The model under review builds one solid part; all positions refer to its coordinate system, in mm. Face numbers are marked on the shaded views. A direction names the side the tool comes from. Round coordinates to 2 decimals unless told otherwise and drop trailing zeros. Loops run counter-clockwise (first coordinate to the right, second up) from the corner with the lowest first, then second, coordinate; pieces in that order, holes last. Notation, with made-up numbers: (-22.5, -10.75) -> (13.5, -10.75) arc R31 cw to (13.5, 21.25) -> close; hole circle Ø3 at (13.25, 2.5). An arc over 180 degrees is marked (long way). Use a Markdown table: item, result. Add a question column.
1) Wall thickness on probe 1 along Y at (x, z) = (4.5, 0); probe 2 along X at (y, z) = (-10, -8); probe 3 along Y at (x, z) = (9, 0): over which ranges is each line inside the solid? List them lowest first.
2) For the marked faces 1, 2 and 3, list the 3-axis set-ups (+Z, -Z, +X, -X, +Y, -Y) from which the entire face can be reached by the end or side of a thin tool; tool diameter is ignored.
3) Insertion check: pin 1 (13.5 mm diameter, centred on y = 1.5, z = 5.5, fed in from -X); pin 2 (1.5 mm diameter, centred on x = -14, z = -6, fed in from -Y); pin 3 (1 mm diameter, centred on x = 8, y = 3, fed in from +Z). Each pin has a flat end and moves straight along its axis. Give the tip position at first contact, or say it passes through.
4) Consider section A-A on x = 0. Give the boundary of the cut face in (y, z), plus the area to 3 significant figures.
5) Consider section B-B on x = -19.5. Give the boundary of the cut face in (y, z), plus the area to 3 significant figures.
6) Mouldability with a two-part tool opening along Y and no side actions: class the marked faces 4, 5 and 6 as released by +Y, released by -Y, zero draft, split by the parting line, or undercut.
7) Consider section C-C on x = 12. Give the boundary of the cut face in (y, z).
from build123d import *

# Parameters (mm, degrees)
EXTRUDE1_DEPTH     = 32.146875
SKETCH3_OUTSIDE_W  = 278.22
SKETCH3_OUTSIDE_H  = 283.376
SKETCH3_OUTSIDE_R  = 16.66875
CUT_EXTRUDE1_DEPTH = 42.008923024
CUT_EXTRUDE1_DRAFT = -70
SKETCH4_OUTSIDE_W  = 278.22
SKETCH4_OUTSIDE_H  = 283.376
SKETCH4_OUTSIDE_R  = 16.66875
CUT_EXTRUDE2_DEPTH = 42.008923024
CUT_EXTRUDE2_DRAFT = -70
SKETCH5_R          = 10.668
EXTRUDE2_DEPTH     = 19.05
EXTRUDE2_DRAFT     = 1.5
SKETCH7_R          = 13.335
CUT_EXTRUDE4_DEPTH = 46.191749083
CUT_EXTRUDE4_DRAFT = 1.5
SKETCH12_W         = 6.35
SKETCH12_H         = 19.247414599
SKETCH15_R         = 13.926557298
CUT_EXTRUDE7_DEPTH = 5.08
CUT_EXTRUDE7_DRAFT = -45


with BuildPart() as part:
    # Sketch2 → Extrude1 (new body)
    with BuildSketch(Plane(origin=(-25.5984375, 0, 0), x_dir=(0, 0, -1), z_dir=(1, 0, 0))):
        Polygon((0, 19.247414599), (-16.66875, 9.6237073), (-16.66875, -9.6237073), (0, -19.247414599), (16.66875, -9.6237073), (16.66875, 9.6237073), align=None)
    extrude(amount=EXTRUDE1_DEPTH)


with BuildPart() as cut_extrude1_tool:
    # Sketch3 outside → Cut-Extrude1 (with draft: the straight prism first)
    with BuildSketch(Plane(origin=(6.5484375, 0, 0), x_dir=(0, 0, -1), z_dir=(1, 0, 0))):
        Rectangle(SKETCH3_OUTSIDE_W, SKETCH3_OUTSIDE_H)
        Circle(SKETCH3_OUTSIDE_R, mode=Mode.SUBTRACT)
    extrude(amount=-CUT_EXTRUDE1_DEPTH)
    # Cut-Extrude1: the draft: its side faces are tilted about the plane it starts from
    cut_extrude1_sides = [cut_extrude1_tool.faces().sort_by_distance(p)[0] for p in [
        (-14.456024012, -141.688, 0),
        (-14.456024012, 0, -139.11),
        (-14.456024012, 141.688, 0),
        (-14.456024012, 0, 139.11),
        (-14.456024012, 0, 16.66875),
    ]]
    draft(cut_extrude1_sides, Plane(origin=(6.5484375, 0, 0), x_dir=(0, 0, -1), z_dir=(1, 0, 0)), CUT_EXTRUDE1_DRAFT)


with BuildPart() as part_1:
    add(part.part)

    # Cut-Extrude1: cut by cut_extrude1_tool
    add(cut_extrude1_tool.part, mode=Mode.SUBTRACT)


with BuildPart() as cut_extrude2_tool:
    # Sketch4 outside → Cut-Extrude2 (with draft: the straight prism first)
    with BuildSketch(Plane.ZY.offset(25.5984375)):
        Rectangle(SKETCH4_OUTSIDE_W, SKETCH4_OUTSIDE_H)
        Circle(SKETCH4_OUTSIDE_R, mode=Mode.SUBTRACT)
    extrude(amount=-CUT_EXTRUDE2_DEPTH)
    # Cut-Extrude2: the draft: its side faces are tilted about the plane it starts from
    cut_extrude2_sides = [cut_extrude2_tool.faces().sort_by_distance(p)[0] for p in [
        (-4.593975988, -141.688, 0),
        (-4.593975988, 0, 139.11),
        (-4.593975988, 141.688, 0),
        (-4.593975988, 0, -139.11),
        (-4.593975988, 0, -16.66875),
    ]]
    draft(cut_extrude2_sides, Plane.ZY.offset(25.5984375), CUT_EXTRUDE2_DRAFT)


with BuildPart() as part_2:
    add(part_1.part)

    # Cut-Extrude2: cut by cut_extrude2_tool
    add(cut_extrude2_tool.part, mode=Mode.SUBTRACT)


with BuildPart() as body_2:
    # Sketch5 → Extrude2 (with draft: the straight prism first)
    with BuildSketch(Plane(origin=(25.5984375, 0, 0), x_dir=(0, 0, -1), z_dir=(1, 0, 0))):
        Circle(SKETCH5_R)
    extrude(amount=-EXTRUDE2_DEPTH)
    # Extrude2: the draft: its side faces are tilted about the plane it starts from
    extrude2_sides = [body_2.faces().sort_by_distance(p)[0] for p in [
        (16.0734375, 0, 10.668),
    ]]
    draft(extrude2_sides, Plane(origin=(25.5984375, 0, 0), x_dir=(0, 0, -1), z_dir=(1, 0, 0)), EXTRUDE2_DRAFT)

    # Sketch17 → Cut-Revolve2 (revolve, cut)
    with BuildSketch(Plane.XY, mode=Mode.PRIVATE) as cut_revolve2_sk:
        Polygon((25.5984375, 10.979645334), (25.5984375, 9.108586861), (23.727379027, 10.979645334), align=None)
        Polygon((6.5484375, 9.853808667), (7.8184375, 9.853808667), (9.325274167, 11.360645334), (6.5484375, 11.360645334), align=None)
    revolve(cut_revolve2_sk.sketch.rotate(Axis((-25.5984375, 0, 0), (1, 0, 0)), 270), axis=Axis((-25.5984375, 0, 0), (1, 0, 0)), mode=Mode.SUBTRACT)


with BuildPart() as cut_extrude4_tool:
    # Sketch7 → Cut-Extrude4 (with draft: the straight prism first)
    with BuildSketch(Plane(origin=(-11.7376575, 0, 0), x_dir=(0, 0, -1), z_dir=(1, 0, 0))):
        Circle(SKETCH7_R)
    extrude(amount=-CUT_EXTRUDE4_DEPTH)
    # Cut-Extrude4: the draft: its side faces are tilted about the plane it starts from
    cut_extrude4_sides = [cut_extrude4_tool.faces().sort_by_distance(p)[0] for p in [
        (-34.833532041, 0, 13.335),
    ]]
    draft(cut_extrude4_sides, Plane(origin=(-11.7376575, 0, 0), x_dir=(0, 0, -1), z_dir=(1, 0, 0)), CUT_EXTRUDE4_DRAFT)


with BuildPart() as part_3:
    add(part_2.part)

    # Cut-Extrude4: cut by cut_extrude4_tool
    add(cut_extrude4_tool.part, mode=Mode.SUBTRACT)


with BuildPart() as body_2_1:
    add(body_2.part)

    # Combine1: union part
    add(part_3.part)

    # Sketch12 → Cut-Revolve1 (revolve, cut)
    with BuildSketch(Plane.XY, mode=Mode.PRIVATE) as cut_revolve1_sk:
        Polygon((-11.7376575, 12.745793431), (-11.7376575, 0), (25.5984375, 0), (25.5984375, 6.35), (-5.341864069, 6.35), align=None)
        with Locations((-28.7734375, 9.6237073)):
            Rectangle(SKETCH12_W, SKETCH12_H)
    revolve(cut_revolve1_sk.sketch.rotate(Axis((-25.5984375, 0, 0), (1, 0, 0)), 90), axis=Axis((-25.5984375, 0, 0), (1, 0, 0)), mode=Mode.SUBTRACT)


with BuildPart() as cut_extrude7_tool:
    # Sketch15 → Cut-Extrude7 (with draft: the straight prism first)
    with BuildSketch(Plane.ZY.offset(25.5984375)):
        Circle(SKETCH15_R)
    extrude(amount=-CUT_EXTRUDE7_DEPTH)
    # Cut-Extrude7: the draft: its side faces are tilted about the plane it starts from
    cut_extrude7_sides = [cut_extrude7_tool.faces().sort_by_distance(p)[0] for p in [
        (-23.0584375, 0, -13.926557298),
    ]]
    draft(cut_extrude7_sides, Plane.ZY.offset(25.5984375), CUT_EXTRUDE7_DRAFT)


with BuildPart() as body_2_2:
    add(body_2_1.part)

    # Cut-Extrude7: cut by cut_extrude7_tool
    add(cut_extrude7_tool.part, mode=Mode.SUBTRACT)


solid = body_2_2.part
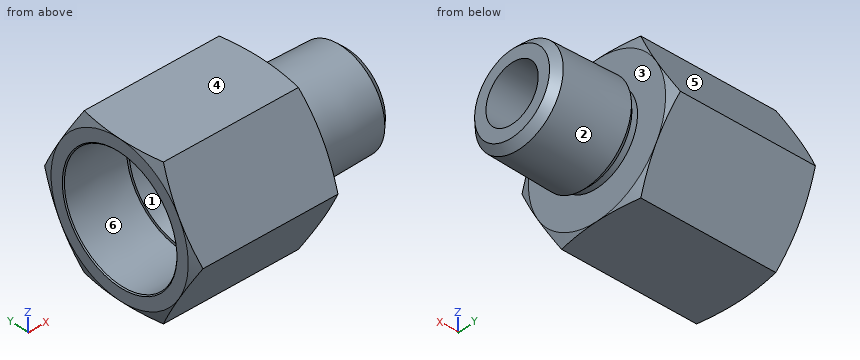
Result set:
| question | item | result |
|---|---|---|
| 1 | probe 1 | -19.25 to -6.35, 6.35 to 19.25 |
| 1 | probe 2 | -11.74 to 6.55 |
| 1 | probe 3 | -11.04 to -6.35, 6.35 to 11.04 |
| 2 | face 1 | -X |
| 2 | face 2 | +X |
| 2 | face 3 | none |
| 3 | pin 1 | x = -11.44 |
| 3 | pin 2 | y = -16.22 |
| 3 | pin 3 | z = 10.12 |
| 4 | outline | (-19.25, 0) -> (-9.62, -16.67) -> (9.62, -16.67) -> (19.25, 0) -> (9.62, 16.67) -> (-9.62, 16.67) -> close; hole circle Ø12.7 at (0, 0) |
| 4 | area | 836 mm2 |
| 5 | outline | (-19.25, 0) -> (-9.62, -16.67) -> (9.62, -16.67) -> (19.25, 0) -> (9.62, 16.67) -> (-9.62, 16.67) -> close; hole circle Ø27.08 at (0, 0) |
| 5 | area | 387 mm2 |
| 6 | face 4 | zero draft |
| 6 | face 5 | released by +Y |
| 6 | face 6 | undercut |
| 7 | outline | circle Ø22.05 at (0, 0); hole circle Ø12.7 at (0, 0) |
